from build123d import *

# Parameters (mm, degrees)
SKETCH3_R                = 35
SKETCH3_R_2              = 20
BOSS_EXTRUDE1_DEPTH      = 30
LPATTERN2_COUNT          = 2
LPATTERN2_PITCH          = 110
BOSS_EXTRUDE2_DEPTH      = 20
BOSS_EXTRUDE2_DEPTH_BACK = 20
FILLET1_R                = 2
BOSS_EXTRUDE3_DEPTH      = 20
BOSS_EXTRUDE3_DEPTH_BACK = 20
SKETCH6_W                = 40
SKETCH6_H                = 30
BOSS_EXTRUDE4_DEPTH      = 14
BOSS_EXTRUDE4_DEPTH_BACK = 14
SKETCH6_3_W              = 28
SKETCH6_3_H              = 70
FILLET2_R                = 14
FILLET3_R                = 20
FILLET4_R                = 5


with BuildPart() as part:
    # Sketch3 → Boss-Extrude1 (new body)
    with BuildSketch(Plane(origin=(0, 0, 0), x_dir=(1, 0, 0), z_dir=(0, 1, 0))):
        with Locations(Location((0, 0, 0), (0, 0, 270))):
            Circle(SKETCH3_R)
        with Locations(Location((0, 0, 0), (0, 0, 270))):
            Circle(SKETCH3_R_2, mode=Mode.SUBTRACT)
    extrude(amount=BOSS_EXTRUDE1_DEPTH)


with BuildPart() as lpattern2_1:
    # LPattern2: pattern copy
    add(part.part.moved(Location(Vector(0, 1, 0) * (1 * LPATTERN2_PITCH))))


with BuildPart() as part_1:
    add(part.part)

    add(lpattern2_1.part)  # Boss-Extrude2 merges LPattern2_1
    # Sketch5 → Boss-Extrude2 (add, two sides: drawn at the far end of the back side and taken through both)
    with BuildSketch(Plane(origin=(0, 0, 0), x_dir=(0, -1, 0), z_dir=(0, 0, 1)).offset(-BOSS_EXTRUDE2_DEPTH_BACK)):
        with BuildLine():
            Line((-10, 21.3), (-10, 50))
            ThreePointArc((-10, 50), (-70, 110), (-130, 50))
            Line((-130, 50), (-130, 21.3))
            Line((-130, 21.3), (-110, 21.3))
            Line((-110, 21.3), (-110, 50))
            ThreePointArc((-110, 50), (-70, 90), (-30, 50))
            Line((-30, 50), (-30, 21.3))
            Line((-30, 21.3), (-10, 21.3))
        make_face()
    extrude(amount=BOSS_EXTRUDE2_DEPTH + BOSS_EXTRUDE2_DEPTH_BACK)

    # Fillet1
    fillet1_edges = [part_1.edges().sort_by_distance(p)[0] for p in [
        (35, 10, 0),
        (35, 130, 0),
    ]]
    fillet(fillet1_edges, radius=FILLET1_R)

    # Sketch6 → Boss-Extrude3 (add, two sides: drawn at the far end of the back side and taken through both)
    with BuildSketch(Plane(origin=(0, 0, 0), x_dir=(0, -1, 0), z_dir=(0, 0, 1)).offset(-BOSS_EXTRUDE3_DEPTH_BACK)):
        with Locations((-70, 115)):
            Rectangle(SKETCH6_W, SKETCH6_H)
    extrude(amount=BOSS_EXTRUDE3_DEPTH + BOSS_EXTRUDE3_DEPTH_BACK)

    # Sketch6<3> → Boss-Extrude4 (add, two sides: drawn at the far end of the back side and taken through both)
    with BuildSketch(Plane(origin=(0, 0, 0), x_dir=(0, -1, 0), z_dir=(0, 0, 1)).offset(-BOSS_EXTRUDE4_DEPTH_BACK)):
        with Locations((-70, 165)):
            Rectangle(SKETCH6_3_W, SKETCH6_3_H)
    extrude(amount=BOSS_EXTRUDE4_DEPTH + BOSS_EXTRUDE4_DEPTH_BACK)

    # Fillet2
    fillet2_edges = [part_1.edges().sort_by_distance(p)[0] for p in [
        (165, 56, -14),
        (165, 56, 14),
        (165, 84, 14),
        (165, 84, -14),
    ]]
    fillet(fillet2_edges, radius=FILLET2_R - 0.0001)  # a hair under: the kernel refuses the full size

    # Fillet3
    fillet3_edges = [part_1.edges().sort_by_distance(p)[0] for p in [
        (118.284271247, 50, -20),
        (118.284271247, 50, 20),
        (118.284271247, 90, 20),
        (118.284271247, 90, -20),
    ]]
    fillet(fillet3_edges, radius=FILLET3_R - 0.0001)  # a hair under: the kernel refuses the full size

    # Fillet4
    fillet4_edges = [part_1.edges().sort_by_distance(p)[0] for p in [
        (130, 60.100475774, -9.899524226),
        (130, 60.100475774, 9.899524226),
        (130, 79.899524226, 9.899524226),
        (130, 79.899524226, -9.899524226),
    ]]
    fillet(fillet4_edges, radius=FILLET4_R)


solid = part_1.part
CAD build for the part. Positions are in the model's coordinates, mm. A direction names the side the tool comes from. Give positions to 0.01 mm unless a question says otherwise; leave off trailing zeros. Write each loop counter-clockwise with the first axis right and the second up, starting at its lowest first coordinate (ties: lowest second). Pieces come first, ordered by that corner, then holes. Notation, with made-up numbers: (60.25, -19) - (79.25, -19) arc R17 ccw to (79.25, -6) - close; hole circle Ø4 at (35.25, -35). An arc over 180 degrees is marked (long way). Put each result on its own line as item: value.
(1) Saw through at C-C (y = 117). List the corners of the cut face in (x, z), then the cut area to 3 significant figures.
Working result:
outline: (28.72, -20) - (87.3, -20) - (87.3, 20) - (28.72, 20) arc R35 ccw (long way) to start; hole circle Ø40 at (0, 0)
area: 4,760 mm^2
(2) Saw through at A-A (x = 40). List the corners of the cut face in (y, z), then the cut area to 3 significant figures.
Working result:
outline: (10, -20) - (30, -20) - (30, 20) - (10, 20) - close; (110, -20) - (130, -20) - (130, 20) - (110, 20) - close
area: 1,600 mm^2
(3) Tool access for faces 4 (the cylindrical face through (-19.524, 124.79, -4.336)), 5 (the flat face through (130, 52, 7)), 6 (the cylindrical face through (118.448, 56.014, -14.297)), 7 (the cylindrical face through (118.448, 56.014, 14.297)), 8 (the cylindrical face through (118.448, 84.297, 13.986)): list every direction of +Z, -Z, +X, -X, +Y, -Y with a clear straight run to the whole face (end or side of a thin tool).
Working result:
face 4: +Y, -Y
face 5: +X
face 6: -Z, +X, -Y
face 7: +Z, +X, -Y
face 8: +Z, +X, +Y
(4) Drop flat-ended pins along their axis: pin 1 Ø15 at (x, z) = (45, 3) entering from +Y; pin 2 Ø15 at (x, z) = (41, 8) entering from -Y; pin 3 Ø8 at (x, z) = (155, 4.5) entering from +Y; pin 4 Ø3 at (x, y) = (147.5, 74) entering from -Z (3 decimals). Give the stop position or say it passes through.
Working result:
pin 1: y = 130
pin 2: y = 0
pin 3: y = 83.99
pin 4: z = -13.775
(5) Pull direction X, two halves, no side cores. Call faces 1 (the cylindrical face through (-34.168, 14.79, -7.587)), 2 (the cylindrical face through (-19.524, 14.79, -4.336)), 3 (the cylindrical face through (168, 80, -9.8)): released by +X, released by -X, zero draft, split by the parting line, or undercut.
Working result:
face 1: split by the parting line
face 2: undercut
face 3: zero draft
(6) Saw through at D-D (z = -7). Count the separate pieces of the cut face and the enclosed holes in it, then the cut area to 3 significant figures.
Working result:
separate pieces: 3
enclosed holes: 0
area: 8,130 mm^2
(7) Saw through at B-B (x = 0). List the corners of the cut face in (y, z).
Working result:
outline: (0, -35) - (30, -35) - (30, -20) - (0, -20) - close; (0, 20) - (30, 20) - (30, 35) - (0, 35) - close; (110, -35) - (140, -35) - (140, -20) - (110, -20) - close; (110, 20) - (140, 20) - (140, 35) - (110, 35) - close
(8) Wall check: L1, parallel to Y at x = 37.5, z = 15; L2, parallel to Y at x = 0, z = 21; L3, parallel to X at y = 8.25, z = 0. Give the ranges that are in metal, low to high.
Working result:
L1: 10 to 30, 110 to 130
L2: 0 to 30, 110 to 140
L3: -35 to -20, 20 to 35.02
